For this review, take the finished solid that the model builds, in its own axes (mm). Face numbers are marked on the shaded views. A direction names the side the tool comes from. Coordinates: 2 decimals unless noted, no trailing zeros. Write each loop counter-clockwise with the first axis right and the second up, starting at its lowest first coordinate (ties: lowest second). Pieces come first, ordered by that corner, then holes.
1) We need section D-D on x = 12. Write out the cut boundary in (y, z), then the cut area to 3 significant figures.
2) For the marked faces 4 and 5, list the 3-axis set-ups (+Z, -Z, +X, -X, +Y, -Y) from which the entire face can be reached by the end or side of a thin tool; tool diameter is ignored.
3) Mouldability with a two-part tool opening along X and no side actions: class the marked faces 1, 2 and 3 as pulls with the +X half, pulls with the -X half, needs draft (parallel to the pull), parting line crosses it, or undercut.
4) We need section B-B on z = -10. Write out the cut boundary in (x, y).
5) We need section C-C on y = 10. Write out the cut boundary in (x, z), then the cut area to 3 significant figures.
6) To check wall thickness, follow line 1 along X through (y, z) = (1.3, -10); line 2 along Z through (x, y) = (9, 1.25); line 3 along X through (y, z) = (20.5, -11). State the ranges of each line that lie inside material, in increasing order.
7) We need section A-A on x = 77. Write out the cut boundary in (y, z).
8) Insertion check: P1, Ø3, axis at x = 49.5, z = -31.5, coming from the +Y side; P2, Ø2.5, axis at x = 9, z = -10, coming from the -Y side. Each pin has a flat end and moves straight along its axis. Give the tip position at first contact, or say it passes through.
from build123d import *

# Parameters (mm, degrees)
SKETCH1_W           = 86
SKETCH1_H           = 42
SKETCH1_R           = 1.5
BOSS_EXTRUDE1_DEPTH = 35
FILLET1_R           = 3
CUT_EXTRUDE1_DEPTH  = 33


with BuildPart() as part:
    # Sketch1 → Boss-Extrude1 (new body)
    with BuildSketch(Plane(origin=(0, 0, 0), x_dir=(1, 0, 0), z_dir=(0, 1, 0))):
        with Locations((43, 21)):
            Rectangle(SKETCH1_W, SKETCH1_H)
        with Locations((9, 10)):
            Circle(SKETCH1_R, mode=Mode.SUBTRACT)
        with Locations((77, 10)):
            Circle(SKETCH1_R, mode=Mode.SUBTRACT)
    extrude(amount=BOSS_EXTRUDE1_DEPTH)

    # Fillet1
    fillet1_edges = [part.edges().sort_by_distance(p)[0] for p in [
        (0, 17.5, -42),
        (86, 17.5, -42),
        (86, 17.5, 0),
        (0, 17.5, 0),
    ]]
    fillet(fillet1_edges, radius=FILLET1_R)

    # Sketch2 → Cut-Extrude1 (cut)
    with BuildSketch(Plane(origin=(0, 35, 0), x_dir=(1, 0, 0), z_dir=(0, 1, 0))):
        with BuildLine():
            Line((6.7, 3.7), (79.3, 3.7))
            ThreePointArc((79.3, 3.7), (81.421320344, 4.578679656), (82.3, 6.7))
            Line((82.3, 6.7), (82.3, 35.3))
            ThreePointArc((82.3, 35.3), (81.421320344, 37.421320344), (79.3, 38.3))
            Line((79.3, 38.3), (6.7, 38.3))
            ThreePointArc((6.7, 38.3), (4.578679656, 37.421320344), (3.7, 35.3))
            Line((3.7, 35.3), (3.7, 6.7))
            ThreePointArc((3.7, 6.7), (4.578679656, 4.578679656), (6.7, 3.7))
        make_face()
    extrude(amount=-CUT_EXTRUDE1_DEPTH, mode=Mode.SUBTRACT)


solid = part.part
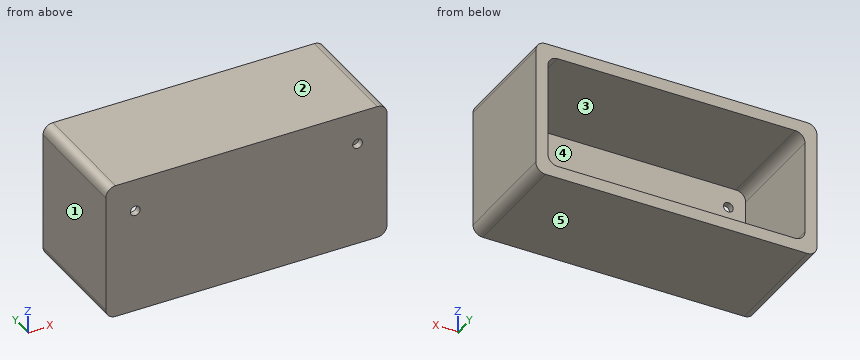
Result:
1. outline: (0, -42) - (35, -42) - (35, -38.3) - (2, -38.3) - (2, -3.7) - (35, -3.7) - (35, 0) - (0, 0) - close
1. area: 328 mm2
2. face 4: +Y
2. face 5: -Z, +X, -X, +Y, -Y
3. face 1: pulls with the -X half
3. face 2: needs draft
3. face 3: undercut
4. outline: (0, 0) - (7.5, 0) - (7.5, 2) - (3.7, 2) - (3.7, 35) - (0, 35) - close; (10.5, 0) - (75.5, 0) - (75.5, 2) - (10.5, 2) - close; (78.5, 0) - (86, 0) - (86, 35) - (82.3, 35) - (82.3, 2) - (78.5, 2) - close
5. outline: (0, -39) arc R3 ccw to (3, -42) - (83, -42) arc R3 ccw to (86, -39) - (86, -3) arc R3 ccw to (83, 0) - (3, 0) arc R3 ccw to (0, -3) - close; hole (3.7, -35.3) arc R3 ccw to (6.7, -38.3) - (79.3, -38.3) arc R3 ccw to (82.3, -35.3) - (82.3, -6.7) arc R3 ccw to (79.3, -3.7) - (6.7, -3.7) arc R3 ccw to (3.7, -6.7) - close
5. area: 892 mm2
6. line 1: x = 0 to 7.5, 10.5 to 75.5, 78.5 to 86
6. line 2: z = -42 to -11.5, -8.5 to 0
6. line 3: x = 0 to 3.7, 82.3 to 86
7. outline: (0, -42) - (35, -42) - (35, -38.3) - (2, -38.3) - (2, -11.5) - (0, -11.5) - close; (0, -8.5) - (2, -8.5) - (2, -3.7) - (35, -3.7) - (35, 0) - (0, 0) - close
8. P1: stops at y = 2
8. P2: passes through
